```python
from build123d import *

# Parameters (mm, degrees)
SKETCH_1_W                  = 30
SKETCH_1_H                  = 24
EXTRUDE_1_DEPTH             = 5
SKETCH_2_W                  = 5
SKETCH_2_H                  = 24
EXTRUDE_2_DEPTH             = 20
EXTRUDE_3_DEPTH             = 24
SKETCH_4_R                  = 2.6
CUT_EXTRUDE_1_DEPTH         = 47.389654019
EXTRUDE_4_DEPTH             = 12
EXTRUDE_4_DIRECTION_2_REACH = 48.39
SKETCH_6_W                  = 14
SKETCH_6_H                  = 8
CUT_EXTRUDE_2_DEPTH         = 9
SKETCH_7_R                  = 1.6
CUT_EXTRUDE_3_DEPTH         = 64.955062348
CUT_EXTRUDE_4_DEPTH         = 2.6
SKETCH_10_R                 = 6
EXTRUDE_5_DEPTH             = 1
FILLET_1_R                  = 2.5
FILLET_2_R                  = 2.5
CHAMFER_1_SIZE              = 1


with BuildPart() as part:
    # Эскиз1 → Бобышка-Вытянуть1 (new body)
    with BuildSketch(Plane.XY):
        with Locations((15, -12)):
            Rectangle(SKETCH_1_W, SKETCH_1_H)
    extrude(amount=EXTRUDE_1_DEPTH)

    # Эскиз2 → Бобышка-Вытянуть2 (add)
    with BuildSketch(Plane.XY.offset(5)):
        with Locations((2.5, -12)):
            Rectangle(SKETCH_2_W, SKETCH_2_H)
        with Locations((27.5, -12)):
            Rectangle(SKETCH_2_W, SKETCH_2_H)
    extrude(amount=EXTRUDE_2_DEPTH)

    # Эскиз3 → Бобышка-Вытянуть3 (add)
    with BuildSketch(Plane(origin=(0, 0, 0), x_dir=(1, 0, 0), z_dir=(0, 1, 0))):
        Polygon((25.2, -25), (25.2, -26), (26.4, -26), (27.4, -25), align=None)
        Polygon((4.8, -25), (4.8, -26), (3.6, -26), (2.6, -25), align=None)
    extrude(amount=-EXTRUDE_3_DEPTH)

    # Эскиз4 → Вырез-Вытянуть1 (cut, through all)
    with BuildSketch(Plane(origin=(0, 0, 0), x_dir=(-1, 0, 0), z_dir=(0, 0, -1))):
        with Locations((-15, -14)):
            Circle(SKETCH_4_R)
    extrude(amount=-CUT_EXTRUDE_1_DEPTH, mode=Mode.SUBTRACT)

    # Эскиз5 → Бобышка-Вытянуть4 (add)
    with BuildSketch(Plane(origin=(0, 0, 0), x_dir=(-1, 0, 0), z_dir=(0, 0, -1))):
        with BuildLine():
            Line((-22, 0), (-41.5, 0))
            ThreePointArc((-41.5, 0), (-45.5, -4), (-41.5, -8))
            Line((-41.5, -8), (-22, -8))
            ThreePointArc((-22, -8), (-18, -4), (-22, 0))
        make_face()
    extrude(amount=EXTRUDE_4_DEPTH)

    # Бобышка-Вытянуть4 direction 2: up to this face of the body (flat: up to its plane)
    extrude_4_direction_2_end = Plane(part.part.faces().sort_by_distance((5.312409987, -12, 5))[0])
    # Эскиз5 → Бобышка-Вытянуть4 direction 2 (add, up to the picked face)
    with BuildSketch(Plane(origin=(0, 0, 0), x_dir=(-1, 0, 0), z_dir=(0, 0, -1)), mode=Mode.PRIVATE) as extrude_4_direction_2_sk1:
        with BuildLine():
            Line((-22, 0), (-41.5, 0))
            ThreePointArc((-41.5, 0), (-45.5, -4), (-41.5, -8))
            Line((-41.5, -8), (-22, -8))
            ThreePointArc((-22, -8), (-18, -4), (-22, 0))
        make_face()
    extrude_4_direction_2_tool1 = split(extrude(extrude_4_direction_2_sk1.sketch, amount=-EXTRUDE_4_DIRECTION_2_REACH, mode=Mode.PRIVATE), bisect_by=extrude_4_direction_2_end, keep=Keep.BOTH, mode=Mode.PRIVATE)
    add(extrude_4_direction_2_tool1.solids().sort_by(Axis((31.75, -4, 0), (0, 0, 1)))[0])

    # Эскиз6 → Вырез-Вытянуть2 (cut)
    with BuildSketch(Plane(origin=(0, 0, -12), x_dir=(-1, 0, 0), z_dir=(0, 0, -1))):
        with Locations((-31.75, -4)):
            Rectangle(SKETCH_6_W, SKETCH_6_H)
    extrude(amount=-CUT_EXTRUDE_2_DEPTH, mode=Mode.SUBTRACT)

    # Эскиз7 → Вырез-Вытянуть3 (cut, through all)
    with BuildSketch(Plane(origin=(0, 0, -12), x_dir=(-1, 0, 0), z_dir=(0, 0, -1))):
        with Locations((-22, -4)):
            Circle(SKETCH_7_R)
        with Locations((-41.5, -4)):
            Circle(SKETCH_7_R)
    extrude(amount=-CUT_EXTRUDE_3_DEPTH, mode=Mode.SUBTRACT)

    # Эскиз8 → Вырез-Вытянуть4 (cut)
    with BuildSketch(Plane.XY.offset(5)):
        Polygon((41.5, -0.766838493), (38.7, -2.383419246), (38.7, -5.616580754), (41.5, -7.233161507), (44.3, -5.616580754), (44.3, -2.383419246), align=None)
        Polygon((22, -0.766838493), (19.2, -2.383419246), (19.2, -5.616580754), (22, -7.233161507), (24.8, -5.616580754), (24.8, -2.383419246), align=None)
    extrude(amount=-CUT_EXTRUDE_4_DEPTH, mode=Mode.SUBTRACT)

    # Эскиз10 → Бобышка-Вытянуть5 (add)
    with BuildSketch(Plane(origin=(0, 0, 0), x_dir=(-1, 0, 0), z_dir=(0, 0, -1))):
        with Locations(Location((-15, -14, 0), (0, 0, 180))):
            Circle(SKETCH_10_R)
        Polygon((-15, -18.734272207), (-10.9, -16.367136104), (-10.9, -11.632863896), (-15, -9.265727793), (-19.1, -11.632863896), (-19.1, -16.367136104), align=None, mode=Mode.SUBTRACT)
    extrude(amount=EXTRUDE_5_DEPTH)

    # Скругление1
    fillet_1_edges = [part.edges().sort_by_distance(p)[0] for p in [
        (0, 0, 12.5),
        (30, 0, 15),
        (30, -24, 12.5),
        (0, -24, 12.5),
    ]]
    fillet(fillet_1_edges, radius=FILLET_1_R)

    # Скругление2
    fillet_2_edges = [part.edges().sort_by_distance(p)[0] for p in [
        (30, -8, 2.5),
    ]]
    fillet(fillet_2_edges, radius=FILLET_2_R)

    # Фаска1
    chamfer_1_edges = [part.edges().sort_by_distance(p)[0] for p in [
        (9, -14, 0),
    ]]
    chamfer(chamfer_1_edges, length=CHAMFER_1_SIZE - 0.0001)  # a hair under: the kernel refuses the full size


solid = part.part
```
Build history of the part. All positions in model axes, mm. A direction names the side the tool comes from. Coordinates: 2 decimals unless noted, no trailing zeros. Write each loop counter-clockwise with the first axis right and the second up, starting at its lowest first coordinate (ties: lowest second). Pieces come first, ordered by that corner, then holes.
1. Band-saw the part on D-D, the plane y = -4. Give the number of separate pieces and of enclosed holes in the cut face, and give its area (3 significant figures).
Answer block:
separate pieces: 3
enclosed holes: 0
area: 514 mm2
2. Drill centre lines: probe 1 along X at (y, z) = (-16.25, 18); probe 2 along Y at (x, z) = (15, 2.1); probe 3 along X at (y, z) = (-5.25, 1). Where is each one in solid material? Low to high.
Answer block:
probe 1: x = 0 to 5, 25 to 30
probe 2: y = -24 to -16.6, -11.4 to 0
probe 3: x = 0 to 21, 23 to 40.5, 42.5 to 45.3
3. Band-saw the part on B-B, the plane z = 12.5. Give the cut face in (x, y).
Answer block:
outline: (0, -21.5) arc R2.5 ccw to (2.5, -24) - (5, -24) - (5, 0) - (2.5, 0) arc R2.5 ccw to (0, -2.5) - close; (25, -24) - (27.5, -24) arc R2.5 ccw to (30, -21.5) - (30, -2.5) arc R2.5 ccw to (27.5, 0) - (25, 0) - close
4. 3-axis set-ups, long thin cutter, end or side, ignore diameter. For faces 5 (the flat face through (19.1, -14, -0.5)), 6 (the flat face through (34, -8, -1)), 7 (the flat face through (24.75, -4, -8)): which of +Z, -Z, +X, -X, +Y, -Y reach the whole face in a straight line?
Answer block:
face 5: -Z
face 6: -Z, +X, -Y
face 7: -Z, +Y, -Y
5. Pull direction Y, two halves, no side cores. Call faces 1 (the flat face through (20.58, -6.414, 3.718)), 2 (the flat face through (29, -12, 25)), 3 (the cylindrical face through (0.752, -0.713, 12.325)), 4 (the flat face through (17.079, -17.534, -0.493)): released by +Y, released by -Y, zero draft, split by the parting line, or undercut.
Answer block:
face 1: undercut
face 2: zero draft
face 3: released by +Y
face 4: undercut
6. Band-saw the part on C-C, the plane x = 23. Give the cut face in (y, z).
Answer block:
outline: (-24, 0) - (-8, 0) - (-8, -12) - (-5.25, -12) - (-5.25, 2.4) - (-6.66, 2.4) - (-6.66, 5) - (-24, 5) - close; (-2.75, -12) - (0, -12) - (0, 5) - (-1.34, 5) - (-1.34, 2.4) - (-2.75, 2.4) - close
7. Drop flat-ended pins along their axis: pin 1 (2 mm diameter, centred on x = 17.5, y = -8, fed in from +Z); pin 2 (8 mm diameter, centred on x = 29, y = -18.5, fed in from -Z); pin 3 (4.5 mm diameter, centred on x = 15, y = -14, fed in from +Z); pin 4 (1.5 mm diameter, centred on x = 31.5, z = -2.5, fed in from -Y). Give the stop position or say it passes through.
Answer block:
pin 1: stops at z = 5
pin 2: stops at z = 0
pin 3: passes through
pin 4: stops at y = -8
